Study the drawing (mm; zero at the part's minimum x, y, z) and answer. A direction names the side the tool comes from. Coordinates: 2 decimals unless noted, no trailing zeros. Order: outer loops, then holes, each group sorted by start corner. A loop starts at its lowest first (then second) coordinate and runs counter-clockwise, first axis right, second up. Notation, with made-up numbers: (-8, 7) -> (2, 7) arc R20 cw to (2, 16) -> close; hole circle Ø8 at (62.25, 7). An arc over 180 degrees is marked (long way). One line per question, with ' | ' between items.
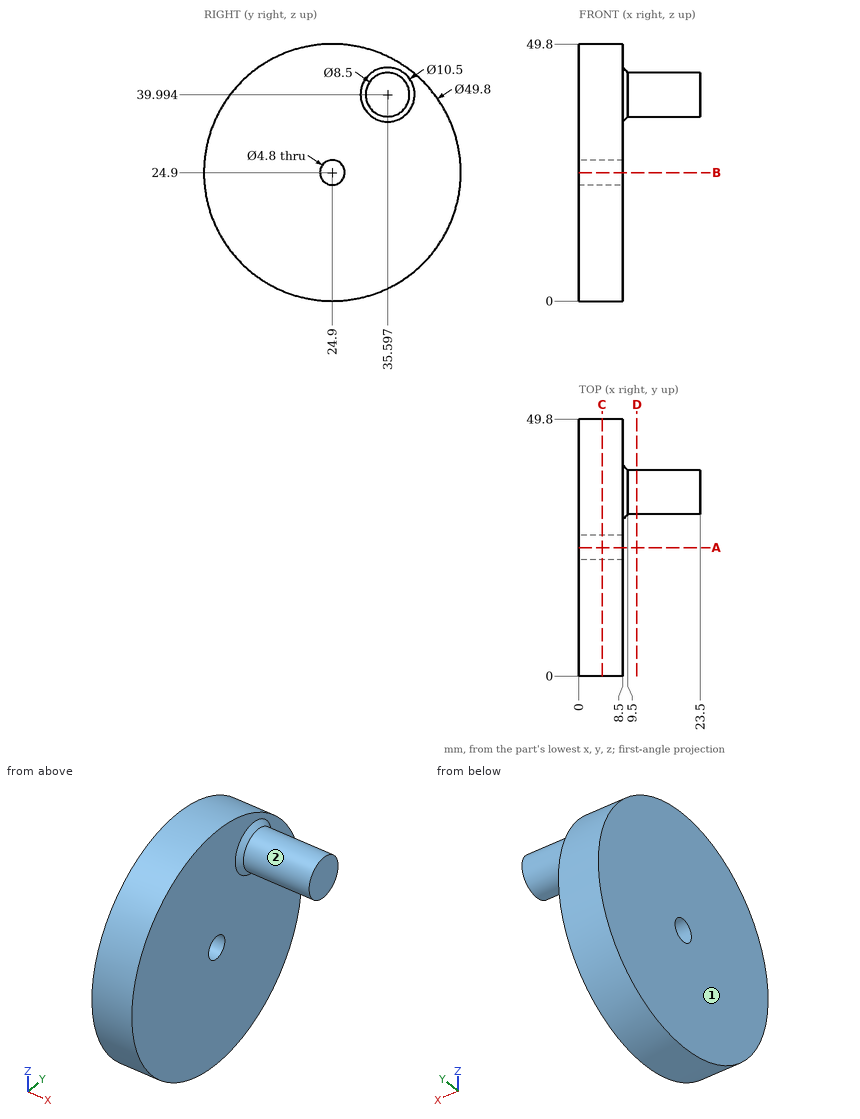
Item 1: Find the intervals of material crossed by L1, parallel to Y at x = 2.25, z = 24.9; L2, parallel to X at y = 30, z = 18; L3, parallel to Z at x = 2.25, y = 32, in increasing order.
Computed values:
L1: y = 0 to 22.5, 27.3 to 49.8 | L2: x = 0 to 8.5 | L3: z = 1.03 to 48.77
Item 2: Section A-A, the plane y = 24.9 is taken. Give the vertices of the cut face in (x, z), plus the area to 4 significant figures.
Computed values:
outline: (0, 0) -> (8.5, 0) -> (8.5, 22.5) -> (0, 22.5) -> close; (0, 27.3) -> (8.5, 27.3) -> (8.5, 49.8) -> (0, 49.8) -> close | area: 382.5 mm^2
Item 3: Section D-D, the plane x = 11.25 is taken. Give the vertices of the cut face in (y, z).
Computed values:
outline: circle Ø8.5 at (35.6, 39.99)
Item 4: Section C-C, the plane x = 4.5 is taken. Give the vertices of the cut face in (y, z).
Computed values:
outline: circle Ø49.8 at (24.9, 24.9); hole circle Ø4.8 at (24.9, 24.9)
Item 5: For the marked faces 1 and 2, determine the directions among +Z, -Z, +X, -X, +Y, -Y from which every point of the face is accessible in a straight line to the end or side of a thin tool.
Computed values:
face 1: +Z, -Z, -X, +Y, -Y | face 2: +X
Item 6: Each of these flat-tipped pins is pushed along its axis until it touches: pin 1 Ø4 at (y, z) = (7, 17.5) entering from -X; pin 2 Ø5.5 at (y, z) = (24.9, 24.9) entering from +X; pin 3 Ø1 at (y, z) = (42.5, 6.5) entering from -X; pin 4 Ø12 at (x, y) = (9, 39.5) entering from -Z. Where does it stop, or does it pass through?
Computed values:
pin 1: stops at x = 0 | pin 2: stops at x = 8.5 | pin 3: passes through | pin 4: stops at z = 1.54
